Design review of the part built by this model. Coordinates are the model's own, in mm. A direction names the side the tool comes from. Coordinates: 2 decimals unless noted, no trailing zeros. Write each loop counter-clockwise with the first axis right and the second up, starting at its lowest first coordinate (ties: lowest second). Pieces come first, ordered by that corner, then holes. Notation, with made-up numbers: (84.25, 83) -> (97.25, 83) arc R28 cw to (97.25, 102) -> close; hole circle Ø2 at (0, -21.75). An arc over 180 degrees is marked (long way). Answer in a Markdown table with one row per item. Add a question column.
Item 1: Take a section at B-B, the plane y = -5. Write out the cut boundary in (x, z) (1 decimal), and give its area (3 significant figures).
Item 2: Take a section at A-A, the plane z = 21.25. Write out the cut boundary in (x, y), and give its area (3 significant figures).
Item 3: To check wall thickness, follow line 1 (Y direction, x = 10.5, z = 2); line 2 (X direction, y = -15, z = 11); line 3 (Z direction, x = 15.5, y = -4). State the ranges of each line that lie inside material, in increasing order.
Item 4: Take a section at C-C, the plane x = -2.75. Write out the cut boundary in (y, z).
Item 5: Draft analysis for pull direction X (two halves, no side actions). For faces 4 (the face through (5, -7, 1.588)), 5 (the face through (-6.39, -12.31, 23.82)), 6 (the face through (18.231, -8, 13)), state which applies: released by +X, released by -X, zero draft, split by the parting line, or undercut.
Item 6: For faces 1 (the face through (-6, -8, 22.225)), 2 (the face through (16.643, -8, 14)), 3 (the face through (5, -19, 25.4)), list the 3-axis set-ups (+Z, -Z, +X, -X, +Y, -Y) from which the entire face can be reached by the end or side of a thin tool; tool diameter is ignored.
Item 7: Clearance check with flat-ended pins moving along their axes: P1, Ø8, axis at x = 4.5, y = -5.5, coming from the +Z side; P2, Ø0.8, axis at x = 18, y = -7, coming from the +Z side (3 decimals). State where each tip first meets the part, or that it passes through.
from build123d import *

# Parameters (mm, degrees)
F0_W      = 25.4
F0_H      = 25.4
F1_DEPTH  = 1.5875
F2_W      = 25.4
F2_H      = 25.4
F3_DEPTH  = 1.5875
F4_W      = 25.4
F4_H      = 25.4
F5_DEPTH  = 1.5875
F7_DEPTH  = 1.5875
F9_DEPTH  = 1.5875
F10_DEPTH = 1.5875
F11_R     = 0.508
F12_R     = 0.508
F13_R     = 0.508
F14_R     = 0.508
F15_R     = 0.508
F16_R     = 0.508
F17_R     = 0.508


with BuildPart() as f1:
    # F0 (on Top) → F1 (new body)
    with BuildSketch(Plane.XY):
        with Locations((5.530645, -7.55323)):
            Rectangle(F0_W, F0_H)
    extrude(amount=F1_DEPTH)

    # F2 (on face) → F3 (join)
    with BuildSketch(Plane.XZ.offset(20.25323)):
        with Locations((5.530645, 12.7)):
            Rectangle(F2_W, F2_H)
    extrude(amount=-F3_DEPTH)

    # F4 (on face) → F5 (join)
    with BuildSketch(Plane(origin=(0, 5.14677, 0), x_dir=(-1, 0, 0), z_dir=(0, 1, 0))):
        with Locations((-5.530645, 12.7)):
            Rectangle(F4_W, F4_H)
    extrude(amount=-F5_DEPTH)

    # F6 (on face) → F7 (join)
    with BuildSketch(Plane.YZ.offset(18.230645)):
        Polygon((-20.25323, 25.4), (-20.25323, 0), (5.14677, 0), (5.14677, 25.4), (-4.37823, 25.4), (-1.20323, 22.225), (-13.90323, 22.225), (-10.72823, 25.4), align=None)
    extrude(amount=-F7_DEPTH)

    # F6 (on face) → F9 (join)
    with BuildSketch(Plane.YZ.offset(18.230645)):
        Polygon((-20.25323, 25.4), (-20.25323, 0), (5.14677, 0), (5.14677, 25.4), (-4.37823, 25.4), (-1.20323, 22.225), (-13.90323, 22.225), (-10.72823, 25.4), align=None)
    extrude(amount=-F9_DEPTH)

    # F8 (on face) → F10 (join)
    with BuildSketch(Plane(origin=(-7.169355, 0, 0), x_dir=(0, -1, 0), z_dir=(-1, 0, 0))):
        Polygon((4.37823, 25.4), (-3.55927, 25.4), (-3.55927, 1.5875), (18.66573, 1.5875), (18.66573, 25.4), (10.72823, 25.4), (13.90323, 22.225), (1.20323, 22.225), align=None)
    extrude(amount=-F10_DEPTH)

    # F11
    f11_edges = [f1.edges().sort_by_distance(p)[0] for p in [
        (-6.375605, -1.20323, 22.225),
    ]]
    fillet(f11_edges, radius=F11_R)

    # F12
    f12_edges = [f1.edges().sort_by_distance(p)[0] for p in [
        (-6.375605, -13.90323, 22.225),
    ]]
    fillet(f12_edges, radius=F12_R)

    # F13
    f13_edges = [f1.edges().sort_by_distance(p)[0] for p in [
        (17.436895, -13.90323, 22.225),
    ]]
    fillet(f13_edges, radius=F13_R)

    # F14
    f14_edges = [f1.edges().sort_by_distance(p)[0] for p in [
        (17.436895, -1.20323, 22.225),
    ]]
    fillet(f14_edges, radius=F14_R)

    # F15
    f15_edges = [f1.edges().sort_by_distance(p)[0] for p in [
        (17.436895, -4.37823, 25.4),
    ]]
    fillet(f15_edges, radius=F15_R)

    # F16
    f16_edges = [f1.edges().sort_by_distance(p)[0] for p in [
        (17.436895, -10.72823, 25.4),
    ]]
    fillet(f16_edges, radius=F16_R)

    # F17
    f17_edges = [f1.edges().sort_by_distance(p)[0] for p in [
        (-6.375605, -4.37823, 25.4),
        (-6.375605, -10.72823, 25.4),
    ]]
    fillet(f17_edges, radius=F17_R)


solid = f1.part
Answers:
| question | item | result |
|---|---|---|
| 1 | outline | (-7.2, 0) -> (18.2, 0) -> (18.2, 22.2) -> (16.6, 22.2) -> (16.6, 1.6) -> (-5.6, 1.6) -> (-5.6, 22.2) -> (-7.2, 22.2) -> close |
| 1 | area | 106 mm^2 |
| 2 | outline | (-7.17, -20.25) -> (18.23, -20.25) -> (18.23, 5.15) -> (-7.17, 5.15) -> close; hole (-5.58, -18.67) -> (16.64, -18.67) -> (16.64, 3.56) -> (-5.58, 3.56) -> close |
| 2 | area | 151 mm^2 |
| 3 | line 1 | y = -20.25 to -18.67, 3.56 to 5.15 |
| 3 | line 2 | x = -7.17 to -5.58, 16.64 to 18.23 |
| 3 | line 3 | z = 0 to 1.59 |
| 4 | outline | (-20.25, 0) -> (5.15, 0) -> (5.15, 25.4) -> (3.56, 25.4) -> (3.56, 1.59) -> (-18.67, 1.59) -> (-18.67, 25.4) -> (-20.25, 25.4) -> close |
| 5 | face 4 | undercut |
| 5 | face 5 | zero draft |
| 5 | face 6 | released by +X |
| 6 | face 1 | +X, -X |
| 6 | face 2 | +Z |
| 6 | face 3 | +Z, +X, -X, +Y, -Y |
| 7 | P1 | stops at z = 1.59 |
| 7 | P2 | stops at z = 22.225 |
